from build123d import *

# Parameters (mm, degrees)
F0_R     = 12.7
F1_DEPTH = 19.05
F2_DEPTH = 6.35
F4_DEPTH = 6.35
F6_DEPTH = 25.4


with BuildPart() as f1:
    # F0 (on Top) → F1 (new body)
    with BuildSketch(Plane.XY):
        with BuildLine():
            ThreePointArc((-11.8853662155, -12.7), (6.9216194995, -15.9575409628), (17.3940199516, 0))
            ThreePointArc((17.3940199516, 0), (6.9216194995, 15.9575409628), (-11.8853662155, 12.7))
            ThreePointArc((-11.8853662155, 12.7), (-17.3940199516, 0), (-11.8853662155, -12.7))
        make_face()
        Circle(F0_R, mode=Mode.SUBTRACT)
    extrude(amount=F1_DEPTH)

    # F0 (on Top) → F2 (join)
    with BuildSketch(Plane.XY):
        with BuildLine():
            ThreePointArc((-11.8853662155, -12.7), (-17.3940199516, 0), (-11.8853662155, 12.7))
            Line((-11.8853662155, 12.7), (-46.5966239572, 12.7))
            Line((-46.5966239572, 12.7), (-46.5966239572, -12.7))
            Line((-46.5966239572, -12.7), (-11.8853662155, -12.7))
        make_face()
    extrude(amount=F2_DEPTH)

    # F3 (on face) → F4 (join)
    with BuildSketch(Plane.XY.offset(6.35)):
        with BuildLine():
            Line((-28.9193168283, 6.35), (-28.9193168283, 0))
            Line((-28.9193168283, 0), (-28.9193168283, -6.35))
            Line((-28.9193168283, -6.35), (-16.1934996241, -6.35))
            ThreePointArc((-16.1934996241, -6.35), (-17.3940199516, 0), (-16.1934996241, 6.35))
            Line((-16.1934996241, 6.35), (-28.9193168283, 6.35))
        make_face()
    extrude(amount=F4_DEPTH)

    # F5 (on face) → F6 (cut)
    with BuildSketch(Plane.XZ.offset(6.35)):
        Polygon((-28.9193168283, 12.7), (-28.9193168283, 6.35), (-16.1934996241, 12.7), align=None)
    extrude(amount=-F6_DEPTH, mode=Mode.SUBTRACT)


solid = f1.part
CAD build for the part. Positions are in the model's coordinates, mm. A direction names the side the tool comes from. Coordinates: 2 decimals unless noted, no trailing zeros. Write each loop counter-clockwise with the first axis right and the second up, starting at its lowest first coordinate (ties: lowest second). Pieces come first, ordered by that corner, then holes. Notation, with made-up numbers: (80.5, -33.75) - (96.5, -33.75) arc R4 cw to (96.5, -28.75) - close; hole circle Ø1 at (-39.5, 23.25). An arc over 180 degrees is marked (long way). Use a Markdown table: item, result. Add a question column.
Item 1: Flat gauge pins, fed straight in: pin 1 (6 mm diameter, centred on x = 0.5, y = 10.5, fed in from +Z); pin 2 (7 mm diameter, centred on x = -32, z = 2.5, fed in from -Y); pin 3 (5 mm diameter, centred on x = -7, z = 2.5, fed in from +Y); pin 4 (5 mm diameter, centred on x = -22, z = 8.5, fed in from +Y). Where does each tip first touch, or does it go through?
Item 2: Mould opens along X. For faces 5 (the face through (-2.75, -12.4, 9.39)), 6 (the face through (-46.597, 0, 3)), 7 (the face through (-21, 6.35, 9)) say: pulls with the +X half, pulls with the -X half, needs draft (parallel to the pull), parting line crosses it, or undercut.
Item 3: Band-saw the part on D-D, the plane z = 8.5. Give the cut face in (x, y), and give its area (3 significant figures).
Item 4: Drill centre lines: L1, parallel to Y at x = 0, z = 6.75; L2, parallel to X at y = -1.5, z = 7.25; L3, parallel to Z at x = -34.5, y = -10. Where is each one in solid material? Low to high. Write a range as from..to.
Item 5: Band-saw the part on C-C, the plane z = 5.25. Give the cut face in (x, y).
Item 6: Band-saw the part on B-B, the plane y = -3. Give the cut face in (x, z), and give its area (3 significant figures).
Item 7: Band-saw the part on A-A, the plane x = 0. Give the cut face in (y, z), and give its area (3 significant figures).
Item 8: 3-axis set-ups, long thin cutter, end or side, ignore diameter. For faces 1 (the face through (-29, 12.7, 3)), 2 (the face through (-20, -6.35, 8)), 3 (the face through (-29, -12.7, 3)), 4 (the face through (-22, 0, 0)): which of +Z, -Z, +X, -X, +Y, -Y reach the whole face in a straight line?
Numbers:
| question | item | result |
|---|---|---|
| 1 | pin 1 | z = 19.05 |
| 1 | pin 2 | y = -12.7 |
| 1 | pin 3 | y = 16.8 |
| 1 | pin 4 | y = 12.7 |
| 2 | face 5 | undercut |
| 2 | face 6 | pulls with the -X half |
| 2 | face 7 | needs draft |
| 3 | outline | (-24.61, -6.35) - (-16.19, -6.35) arc R17.39 ccw (long way) to (-16.19, 6.35) - (-24.61, 6.35) - close; hole circle Ø25.4 at (0, 0) |
| 3 | area | 540 mm2 |
| 4 | L1 | -17.39..-12.7, 12.7..17.39 |
| 4 | L2 | -27.12..-12.61, 12.61..17.33 |
| 4 | L3 | 0..6.35 |
| 5 | outline | (-46.6, -12.7) - (-11.89, -12.7) arc R17.39 ccw (long way) to (-11.89, 12.7) - (-46.6, 12.7) - close; hole circle Ø25.4 at (0, 0) |
| 6 | outline | (-46.6, 0) - (-12.34, 0) - (-12.34, 19.05) - (-17.13, 19.05) - (-17.13, 12.7) - (-16.19, 12.7) - (-28.92, 6.35) - (-46.6, 6.35) - close; (12.34, 0) - (17.13, 0) - (17.13, 19.05) - (12.34, 19.05) - close |
| 6 | area | 404 mm2 |
| 7 | outline | (-17.39, 0) - (-12.7, 0) - (-12.7, 19.05) - (-17.39, 19.05) - close; (12.7, 0) - (17.39, 0) - (17.39, 19.05) - (12.7, 19.05) - close |
| 7 | area | 179 mm2 |
| 8 | face 1 | +Z, -Z, -X, +Y |
| 8 | face 2 | +Z, -X, -Y |
| 8 | face 3 | +Z, -Z, -X, -Y |
| 8 | face 4 | -Z, +X, -X, +Y, -Y |
